Input: part model. Units: mm. Frame: model coordinates. Face numbers are marked on the shaded views. A direction names the side the tool comes from. Coordinates: 2 decimals unless noted, no trailing zeros. Loops run counter-clockwise (first coordinate to the right, second up) from the corner with the lowest first, then second, coordinate; pieces in that order, holes last. Notation, with made-up numbers: (62, -33) - (113, -33) arc R23 cw to (113, -10) - close; hole circle Ø7 at (-8.5, 65). An arc over 180 degrees is marked (long way). Use one line per item in the form item = value.
from build123d import *

# Parameters (mm, degrees)
F0_W     = 30
F0_H     = 30
F1_DEPTH = 30
F2_R     = 3
F3_DEPTH = 6
F4_W     = 19
F4_H     = 19
F5_DEPTH = 6
F6_R     = 1.05
F7_DEPTH = 9.3


with BuildPart() as f1:
    # F0 (on Right) → F1 (new body)
    with BuildSketch(Plane.YZ):
        Rectangle(F0_W, F0_H)
    extrude(amount=F1_DEPTH)

    # F2 (on face) → F3 (cut)
    with BuildSketch(Plane(origin=(0, 0, 0), x_dir=(0, -1, 0), z_dir=(-1, 0, 0))):
        Circle(F2_R)
    extrude(amount=-F3_DEPTH, mode=Mode.SUBTRACT)

    # F4 (on face) → F5 (cut)
    with BuildSketch(Plane.XZ.offset(15)):
        with Locations((20.5, 0)):
            Rectangle(F4_W, F4_H)
    extrude(amount=-F5_DEPTH, mode=Mode.SUBTRACT)

    # F6 (on face) → F7 (cut)
    with BuildSketch(Plane.XZ.offset(15)):
        with Locations((20.5, 11.5)):
            Circle(F6_R)
        with Locations((20.5, -11.5)):
            Circle(F6_R)
    extrude(amount=-F7_DEPTH, mode=Mode.SUBTRACT)


solid = f1.part
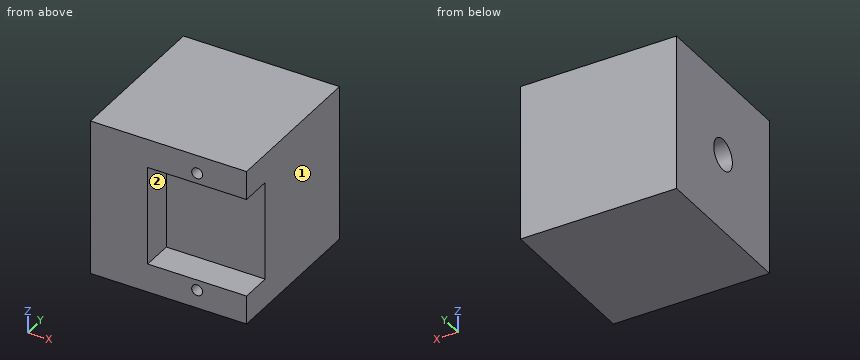
Q1. First-contact query: P1, Ø1, axis at x = 14, z = 7, coming from the -Y side; P2, Ø1.8, axis at y = -0.5, z = -1, coming from the -X side; P3, Ø1.9, axis at x = 20.5, z = 11.5, coming from the -Y side. Flat tips, straight axial feed; report the tip coordinate or a pass-through.
Check values:
P1 = -9
P2 = 6
P3 = -5.7
Q2. Cut plane A-A, the plane y = -11.75. Return loops of the section in (x, z), then the cut area to 3 significant figures.
Check values:
outline = (0, -15) - (30, -15) - (30, -9.5) - (11, -9.5) - (11, 9.5) - (30, 9.5) - (30, 15) - (0, 15) - close; hole circle Ø2.1 at (20.5, -11.5); hole circle Ø2.1 at (20.5, 11.5)
area = 532 mm²
Q3. Cut plane B-B, the plane z = -11.5. Return loops of the section in (x, y), then the cut area to 3 significant figures.
Check values:
outline = (0, -15) - (19.45, -15) - (19.45, -5.7) - (21.55, -5.7) - (21.55, -15) - (30, -15) - (30, 15) - (0, 15) - close
area = 880 mm²
Q4. Cut plane C-C, the plane x = 20.5. Return loops of the section in (y, z).
Check values:
outline = (-15, -15) - (15, -15) - (15, 15) - (-15, 15) - (-15, 12.55) - (-5.7, 12.55) - (-5.7, 10.45) - (-15, 10.45) - (-15, 9.5) - (-9, 9.5) - (-9, -9.5) - (-15, -9.5) - (-15, -10.45) - (-5.7, -10.45) - (-5.7, -12.55) - (-15, -12.55) - close
Q5. Ray query, line 1 along Z through (x, y) = (20.5, -9.25); line 2 along Z through (x, y) = (3.3, 0); line 3 along Y through (x, z) = (17.75, -6.5). Return the intervals inside material, ascending. Write a range as [from, to].
Check values:
line_1 = [-15, -12.55], [-10.45, -9.5], [9.5, 10.45], [12.55, 15]
line_2 = [-15, -3], [3, 15]
line_3 = [-9, 15]
Q6. Set-up query: the marked faces 1 and 2. Return all of +Z, -Z, +X, -X, +Y, -Y with unobstructed straight access to the full face (end or side cutting, diameter ignored); none if empty.
Check values:
face_1 = +Z, -Z, +X, +Y, -Y
face_2 = +X, -Y
Q7. Cut plane D-D, the plane y = 0. Return loops of the section in (x, z).
Check values:
outline = (0, -15) - (30, -15) - (30, 15) - (0, 15) - (0, 3) - (6, 3) - (6, -3) - (0, -3) - close
